Geometry: final body of the model. Coordinates: model frame, mm. Face numbers are marked on the shaded views. A direction names the side the tool comes from. Coordinates: 2 decimals unless noted, no trailing zeros. Order: outer loops, then holes, each group sorted by start corner. A loop starts at its lowest first (then second) coordinate and runs counter-clockwise, first axis right, second up. Notation, with made-up numbers: (46.5, -3.5) -> (84.5, -3.5) arc R24 ccw to (84.5, 13.5) -> close; hole circle Ø11 at (-35.75, 81.25). An arc over 180 degrees is marked (long way). Answer in a Markdown table with one row per item. Add a question column.
1) Section query B-B on z = 13.1. Return the cut outline in (x, y).
2) Section query A-A on x = 9.5. Return the cut outline in (y, z).
3) Contact query for flat-ended pins moving along their axis: P1, Ø1.5, axis at y = 2, z = 3.5, coming from the -X side; P2, Ø1.5, axis at y = 1, z = 1, coming from the +X side; P3, Ø1, axis at x = -5, y = 0.5, coming from the -Z side. Output: stop coordinate, or through.
4) Ray query, line 1 (X direction, y = 2.75, z = 3); line 2 (Z direction, x = -0.5, y = 2.05); line 3 (X direction, y = 2.8, z = -9). Return the intervals inside material, ascending. Write a range as from..to.
5) Section query C-C on y = 1. Count the separate pieces of the cut face and the enclosed holes in it, then the cut area to 3 significant figures.
6) Set-up query: the marked faces 1 and 2. Return all of +Z, -Z, +X, -X, +Y, -Y with unobstructed straight access to the full face (end or side cutting, diameter ignored); none if empty.
7) Pull-direction query (X, two-part tool) for the marked faces 3, 4 and 5; classes: +X half, -X half, draft (parallel to the pull), parting line (faces both ways), or undercut.
Autodesk Inventor part; units mm, degrees
ref_plane "YZ Plane" through (0, 0, 0) normal (1, 0, 0) x (0, 1, 0)
ref_plane "XZ Plane" through (0, 0, 0) normal (0, 1, 0) x (-1, 0, 0)
ref_plane "XY Plane" through (0, 0, 0) normal (0, 0, 1) x (1, 0, 0)
sketch "Эскиз1" plane through (0, 0, 0) normal (0, 1, 0) x (-1, 0, 0)
  line L0 (-7, 13.1) -> (7, 13.1) construction
  line L1 (7, 13.1) -> (7, -13.1) construction
  line L2 (7, -13.1) -> (-7, -13.1) construction
  line L3 (-7, -13.1) -> (-7, 13.1) construction
  line L4 (-7, 13.1) -> (7, -13.1) construction
  line L5 (7, 13.1) -> (-7, -13.1) construction
  line L6 (-1.437822, -16.490381) -> (13.562178, 9.490381) construction
  line L7 (13.562178, 9.490381) -> (1.437822, 16.490381) construction
  line L8 (1.437822, 16.490381) -> (-13.562178, -9.490381) construction
  line L9 (-13.562178, -9.490381) -> (-1.437822, -16.490381) construction
  line L10 (-1.437822, -16.490381) -> (1.437822, 16.490381) construction
  line L11 (13.562178, 9.490381) -> (-13.562178, -9.490381) construction
  circle A0 centre (13.562178, 9.490381) radius 1.5
  circle A1 centre (1.437822, 16.490381) radius 1.5
  circle A2 centre (7, 13.1) radius 1.5
  circle A3 centre (-7, 13.1) radius 1.5
  circle A4 centre (-7, -13.1) radius 1.5
  circle A5 centre (7, -13.1) radius 1.5
  circle A6 centre (-1.437822, -16.490381) radius 1.5
  circle A7 centre (-13.562178, -9.490381) radius 1.5
  circle A8 centre (0, 0) radius 13.352946
  circle A9 centre (0, 0) radius 15.052945
  circle A10 centre (0, 0) radius 18.052945
  circle A11 centre (0, 0) radius 16.352946
  circle A12 centre (0, 0) radius 21.052945
  circle A13 centre (0, 0) radius 10.352946
  line L12 (-2, 10.352946) -> (2, 10.352946) construction
  line L13 (2, 10.352946) -> (2, -10.352946)
  line L14 (2, -10.352946) -> (-2, -10.352946) construction
  line L15 (-2, -10.352946) -> (-2, 10.352946)
  line L16 (-2, 10.352946) -> (2, -10.352946) construction
  line L17 (2, 10.352946) -> (-2, -10.352946) construction
  circle A14 centre (1.157182, 4.993806) radius 10
  circle A15 centre (1.157182, 4.993806) radius 13
  circle A16 centre (5.040606, 1.768152) radius 10
  circle A17 centre (5.040606, 1.768152) radius 13
  circle A18 centre (-1.157182, -4.993806) radius 10
  circle A19 centre (-1.157182, -4.993806) radius 13
  circle A20 centre (-5.040606, -1.768152) radius 10
  circle A21 centre (-5.040606, -1.768152) radius 13
  point P0 (6.29307, 11.77703)
  point P1 (1.307529, 14.996051)
  point P2 (-1.307529, -14.996051)
  point P3 (-6.29307, -11.77703)
  point P4 (-7.70693, -14.42297)
  point P5 (-6.29307, 11.77703)
  point P6 (-7.70693, 14.42297)
  point P7 (14.79116, 10.350383)
  point P8 (12.333196, 8.630379)
  point P9 (6.29307, -11.77703)
  point P10 (7.70693, -14.42297)
  point P11 (-14.79116, -10.350383)
  point P12 (-12.333196, -8.630379)
  point P13 (-2, 10.157927)
  point P14 (-2, -10.157927)
  point P15 (2, -10.157927)
  point P16 (2, 10.157927)
  point P17 (8.377519, -12.506332)
  point P18 (-14.189914, -8.128049)
  point P19 (14.189914, 8.128049)
  point P20 (-8.377519, 12.506332)
  point P21 (7.255573, 14.578067)
  point P22 (14.673687, 10.497628)
  point P23 (12.387672, 8.552003)
  point P24 (6.744427, 11.621933)
  point P25 (6.398093, -8.139281)
  point P26 (6.282627, -8.154417)
  point P27 (6.207779, -8.285346)
  point P28 (8.06398, -14.15733)
  point P29 (-1.474427, -17.989934)
  point P30 (-1.354811, -14.991853)
  point P31 (5.93602, -12.04267)
  point P32 (-7.255573, -14.578067)
  point P33 (-14.673687, -10.497628)
  point P34 (-12.387672, -8.552003)
  point P35 (-6.744427, -11.621933)
  point P36 (1.354811, 14.991853)
  point P37 (-5.93602, 12.04267)
  point P38 (-8.06398, 14.15733)
  point P39 (1.474427, 17.989934)
  dimension "d6" = 3
  dimension "d7" = 3
  dimension "d11" = 3
  dimension "d0" = 14
  dimension "d1" = 26.2
  dimension "d2" = 30
  dimension "d3" = 14
  dimension "d5" = 3
  dimension "d8" = 3
  dimension "d9" = 3
  dimension "d10" = 3
  dimension "d12" = 3
  dimension "d15" = 3
  dimension "d16" = 3
  dimension "d19" = 3
  dimension "d22" = 3
  dimension "d23" = 4
  dimension "d26" = 30
  dimension "d28" = 20
  dimension "d29" = 3
  dimension "d30" = 20
  dimension "d31" = 3
  dimension "d32" = 20
  dimension "d33" = 3
  dimension "d34" = 20
  dimension "d35" = 3
extrude "Выдавливание1" add sketch "Эскиз1" along normal blind 3 contours A0 A10 A17 A11 | A10 A17 | A0 A17 A10 | A11 A17 A9 A16 A15 A0 | A17 A15 A10 | A10 A6 A19 A11 A17 | A15 A16 A0 | A17 A11 A1 A10 A15 | A11 A19 A9 A17 | A10 A1 A15 | A16 A9 A0 | A16 A15 A9 | A16 A9 A15 | A17 A14 A1 A11 | A19 A10 A6 | A17 A19 A8 A16 A9 | A9 A19 A17 | A1 A15 A11 A21 A10 | A9 A15 A8 A14 A16 | A9 A16 A8 A15 | A2 A9 A14 A17 | A10 A19 A21 A11 A6 | A10 A21 A19 | A5 A9 A19 | A9 A5 A8 A17 A19 | A17 A8 A19 | A21 A11 A7 A10 | A10 A21 | A14 A8 A16 | A14 A17 A9 A1 | A2 A14 A9 | A14 A9 A17 | A11 A21 A18 A6 | A10 A7 A21 | A5 A18 A8 | A17 A18 A16 A19 A8 | A8 A18 A17 | A19 A16 A8 | A15 A9 A21 A11 | A21 A9 A20 A19 A7 A11 | A8 A16 A13 A21 A17 | A14 A19 A13 A16 A8 | A8 A15 A19 A14 | A16 A8 A2 | A16 A19 A15 A8 | A9 A17 A8 A14 | A2 A8 A17 A9 A14 | A18 A21 A9 A6 | A18 A9 A21 A8 | A18 A8 A21 A17 | A17 A21 A13 A16 A18 | A16 A18 A15 A19 | A3 A9 A15 | A21 A15 A8 A20 A9 | A9 A15 A21 | A15 A18 A13 A14 A19 | A8 A14 A21 | A8 A21 A15 A9 A3 | A14 A8 A3 | A17 A21 A14 A8 | A21 A4 A9 A18 | A18 A9 A21 | A8 A21 A9 A18 A4 | A21 A8 A20 A13 A17 | A17 A13 A21 | A16 A13 A15 A18 | A19 A20 A7 | A20 A8 A19 A9 | A9 A19 A20 | A21 A8 A15 | A16 A21 A13 | A13 L13 A21 A16 | A14 A13 A19 | A15 A13 A18 | A21 A13 A17 | A17 A13 A20 A14 A21 | A9 A4 A18 | A17 A20 L13 A13 | A13 A20 A17 | A20 A9 A7 | A20 A19 A9 | A19 A8 A18 A20 A9 | A20 A15 A19 A8 | A8 A15 A20 | A8 A21 A14 A20 A15 | A21 A16 L15 A13 | A21 L13 A19 L15 A16 | A4 A20 A8 | A20 A8 A18 A15 A13 | A13 L15 A17 A20 | A17 L15 A15 L13 A20 | A19 A15 A18 A8 | A20 A14 A19 A15 | A20 A13 A19 A14 | A20 A18 A8 | A19 A14 A13 A18 A15 | L13 A20 L15 A19 | A19 A13 A14 | A15 A18 A13 | A15 L15 A16 L13 | L13 A18 L15 A20 | A16 L15 A14 L13 | L13 A14 L15 A18 | A12 picked at (5.651458, 13.934035) picked at (-0.217232, 10.33749) picked at (-5.651458, -13.934035) picked at (0.217232, -10.33749)
fillet "Сопряжение1" radius 2 4 edges at (-2, 1.5, -10.1579) (-2, 1.5, 10.1579) (2, 1.5, 10.1579) (2, 1.5, -10.1579)
sketch "Эскиз2" plane through (0, 3, 0) normal (0, 1, 0) x (1, 0, 0)
  line L0 (-18.777493, -9.520098) -> (-10.754619, 18.098748)
  circle A0 centre (0, 0) radius 21.052945
  line L1 (10.754619, -18.098748) -> (18.777493, 9.520098)
  line L2 (0, 0) -> (0, 4.178964)
  line L3 (-18.777493, -9.520098) -> (10.754619, -18.098748) construction
  arc A1 (-12.333196, -8.630379) -> (-14.673687, -10.497628) centre (-13.562178, -9.490381) ccw
  arc A2 (-8.06398, 14.15733) -> (-5.93602, 12.04267) centre (-7, 13.1) ccw
  dimension "d38" = 5
  dimension "d40" = 5
extrude "Выдавливание2" cut sketch "Эскиз2" against normal blind 3 contours A0 L0 | L1 A0
fillet "Сопряжение2" radius 5 4 edges at (-18.7775, 1.5, 9.5201) (-10.7546, 1.5, -18.0987) (18.7775, 1.5, -9.5201) (10.7546, 1.5, 18.0987)
properties part number "krepezh"
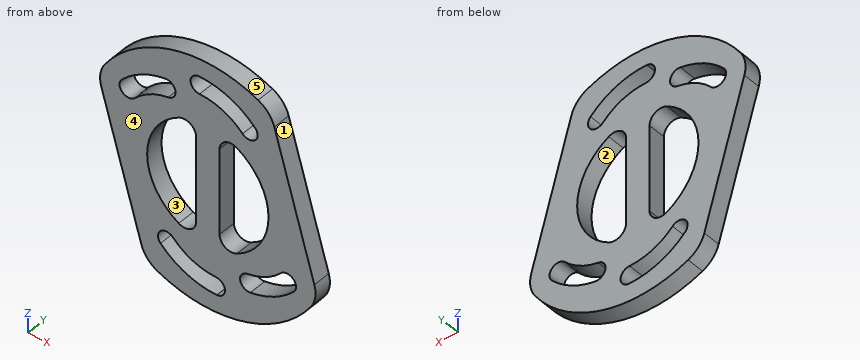
Result:
| question | item | result |
|---|---|---|
| 1 | outline | (-16.48, 0) -> (-11.41, 0) -> (-11.41, 3) -> (-16.48, 3) -> close; (-5.5, 0) -> (4.7, 0) -> (4.7, 3) -> (-5.5, 3) -> close; (8.5, 0) -> (12.21, 0) -> (12.21, 3) -> (8.5, 3) -> close |
| 2 | outline | (0, -18.79) -> (3, -18.79) -> (3, -13.98) -> (0, -13.98) -> close; (0, -10.72) -> (3, -10.72) -> (3, -4.12) -> (0, -4.12) -> close; (0, 4.12) -> (3, 4.12) -> (3, 18.69) -> (0, 18.69) -> close |
| 3 | P1 | x = -17.25 |
| 3 | P2 | x = 15.94 |
| 3 | P3 | z = -20.57 |
| 4 | line 1 | -16.88..-9.91, -2..2, 9.91..15.14 |
| 4 | line 2 | -21.05..-17.89, -14.86..14.97, 17.98..21.05 |
| 4 | line 3 | -13.4..-5.12, -2.9..2.9, 5.12..11.95, 14.98..18.38 |
| 5 | separate pieces | 1 |
| 5 | enclosed holes | 6 |
| 5 | area | 789 mm2 |
| 6 | face 1 | +Z, +X, +Y, -Y |
| 6 | face 2 | +Y, -Y |
| 7 | face 3 | undercut |
| 7 | face 4 | draft |
| 7 | face 5 | parting line |
